```python
from build123d import *

# Parameters (mm, degrees)
BOSS_EXTRUDE1_DEPTH = 250
SKETCH2_W           = 180
SKETCH2_H           = 460
CUT_EXTRUDE1_DEPTH  = 41
SKETCH5_R           = 10
CUT_EXTRUDE5_DEPTH  = 15
SKETCH6_R           = 10
CUT_EXTRUDE6_DEPTH  = 20
SKETCH7_R           = 10
CUT_EXTRUDE7_DEPTH  = 300


with BuildPart() as part:
    # Sketch1 → Boss-Extrude1 (new body, symmetric)
    with BuildSketch(Plane.XY):
        Polygon((-110, 10), (110, 10), (110, 50), (150, 50), (150, 10), (150, -30), (-150, -30), (-150, 10), (-150, 50), (-110, 50), align=None)
    extrude(amount=BOSS_EXTRUDE1_DEPTH, both=True)

    # Sketch2 → Cut-Extrude1 (cut, through all)
    with BuildSketch(Plane(origin=(0, 10, 0), x_dir=(1, 0, 0), z_dir=(0, 1, 0))):
        Rectangle(SKETCH2_W, SKETCH2_H)
    extrude(amount=-CUT_EXTRUDE1_DEPTH, mode=Mode.SUBTRACT)

    # Sketch5 → Cut-Extrude5 (cut)
    with BuildSketch(Plane(origin=(0, 0, 230), x_dir=(-1, 0, 0), z_dir=(0, 0, -1))):
        with Locations((0, -10)):
            Circle(SKETCH5_R)
    extrude(amount=-CUT_EXTRUDE5_DEPTH, mode=Mode.SUBTRACT)

    # Sketch6 → Cut-Extrude6 (cut)
    with BuildSketch(Plane(origin=(0, 0, -250), x_dir=(-1, 0, 0), z_dir=(0, 0, -1))):
        with Locations((0, -10)):
            Circle(SKETCH6_R)
    extrude(amount=-CUT_EXTRUDE6_DEPTH, mode=Mode.SUBTRACT)

    # Sketch7 → Cut-Extrude7 (cut)
    with BuildSketch(Plane.ZY.offset(150)):
        with Locations((0, 35)):
            Circle(SKETCH7_R)
    extrude(amount=-CUT_EXTRUDE7_DEPTH, mode=Mode.SUBTRACT)


solid = part.part
```
Source: CAD feature listing. Evaluate the final solid. Frame: model axes, mm. A direction names the side the tool comes from. Round coordinates to 2 decimals unless told otherwise and drop trailing zeros. Order: outer loops, then holes, each group sorted by start corner. A loop starts at its lowest first (then second) coordinate and runs counter-clockwise, first axis right, second up. Notation, with made-up numbers: (-39, -23.75) -> (-8, -23.75) arc R9 ccw to (-8, -8.75) -> close; hole circle Ø4 at (10, 29). An arc over 180 degrees is marked (long way). One line per item, written item: value. Start each with the question number.
Q1. Material intervals for probe 1 along Z at (x, y) = (52, 4); probe 2 along Y at (x, z) = (0, -236); probe 3 along X at (y, z) = (8.5, 166), sorted ascending.
Q2. Section query D-D (y = -10). Return the cut outline in (x, z), plus the area to 3 significant figures.
Q3. Access query for faces 4 (the cylindrical face through (8, -16, 237)), 5 (the flat face through (-98, 10, 75)), 6 (the flat face through (-1, -23, -230)). Directions: +Z, -Z, +X, -X, +Y, -Y. A direction counts if a zero-diameter tool reaches every point of the face in a straight line with its end or side. Return the directions, or none.
Q4. Draft query along Y for faces 1 (the flat face through (-98, -30, 4)), 2 (the flat face through (-150, 11, 4)), 3 (the cylindrical face through (-130.28, 25.24, -2.17)). Return one class per face: pulls with the +Y half, pulls with the -Y half, needs draft (parallel to the pull), parting line crosses it, or undercut.
Q5. Section query C-C (z = 92). Return the cut outline in (x, y).
Q6. Section query A-A (x = -44.5). Return the cut outline in (y, z), plus the area to 3 significant figures.
Q7. Pin query (flat end, axial travel): pin 1 (16 mm diameter, centred on x = 0, y = -10, fed in from -Z); pin 2 (23 mm diameter, centred on y = 35, z = 0, fed in from +X). Return the tip coordinate at first contact, or that it passes through.
Q8. Section query B-B (z = 0). Return the cut outline in (x, y), plus the area to 3 significant figures.
Findings below:
1. probe 1: -250 to -230, 230 to 250
1. probe 2: -30 to -20, 0 to 10
1. probe 3: -150 to -90, 90 to 150
2. outline: (-150, -250) -> (-10, -250) -> (-10, -230) -> (-90, -230) -> (-90, 230) -> (-10, 230) -> (-10, 245) -> (10, 245) -> (10, 230) -> (90, 230) -> (90, -230) -> (10, -230) -> (10, -250) -> (150, -250) -> (150, 250) -> (-150, 250) -> close
2. area: 66,500 mm²
3. face 4: -Z
3. face 5: +Z, -Z, +Y
3. face 6: +Y, -Y
4. face 1: pulls with the -Y half
4. face 2: needs draft
4. face 3: undercut
5. outline: (-150, -30) -> (-90, -30) -> (-90, 10) -> (-110, 10) -> (-110, 50) -> (-150, 50) -> close; (90, -30) -> (150, -30) -> (150, 50) -> (110, 50) -> (110, 10) -> (90, 10) -> close
6. outline: (-30, -250) -> (10, -250) -> (10, -230) -> (-30, -230) -> close; (-30, 230) -> (10, 230) -> (10, 250) -> (-30, 250) -> close
6. area: 1,600 mm²
7. pin 1: z = 245
7. pin 2: x = 150
8. outline: (-150, -30) -> (-90, -30) -> (-90, 10) -> (-110, 10) -> (-110, 25) -> (-150, 25) -> close; (-150, 45) -> (-110, 45) -> (-110, 50) -> (-150, 50) -> close; (90, -30) -> (150, -30) -> (150, 25) -> (110, 25) -> (110, 10) -> (90, 10) -> close; (110, 45) -> (150, 45) -> (150, 50) -> (110, 50) -> close
8. area: 6,400 mm²
